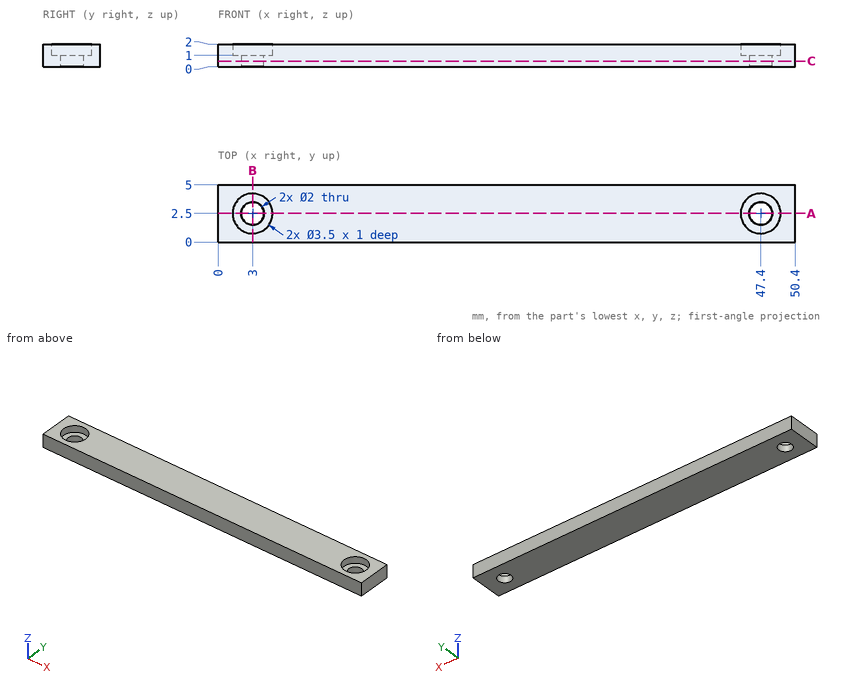
Answer from the drawing. Dimensions are ordinates in mm from the lowest x, y and z of the part. Coordinates: 2 decimals unless noted, no trailing zeros. Write each loop counter-clockwise with the first axis right and the second up, starting at its lowest first coordinate (ties: lowest second). Pieces come first, ordered by that corner, then holes. Notation, with made-up numbers: M -2,-36.5 L 15,-36.5 A29 ccw 15,-10.5 Z; hole C 22.5,80 d5. An arc over 180 degrees is marked long. Write item = value, one per line.
1. Straight lines are drawn through the part: line 1 (X direction, y = 2.5, z = 1.6); line 2 (X direction, y = 2.5, z = 0.65); line 3 (Y direction, x = 3, z = 1.3). For each, find the intervals that lie inside material, in ascending order. Write a range as from..to.
Solution:
line_1 = 0..1.25, 4.75..45.65, 49.15..50.4
line_2 = 0..2, 4..46.4, 48.4..50.4
line_3 = 0..0.75, 4.25..5
2. A flat-ended cylindrical pin translates along its axis: pin 1 (1.2 mm diameter, centred on x = 3, y = 2.5, fed in from +Z). Find the tip coordinate at first contact, or state that the pin passes through.
Solution:
pin_1 = through
3. The part is cut by section B-B (x = 3). Determine the outline of the cut face in (y, z), then the cut area to 3 significant figures.
Solution:
outline = M 0,0 L 1.5,0 L 1.5,1 L 0.75,1 L 0.75,2 L 0,2 Z; M 3.5,0 L 5,0 L 5,2 L 4.25,2 L 4.25,1 L 3.5,1 Z
area = 4.50 mm2
4. The part is cut by section C-C (z = 0.5). Determine the outline of the cut face in (x, y), then the cut area to 3 significant figures.
Solution:
outline = M 0,0 L 50.4,0 L 50.4,5 L 0,5 Z; hole C 3,2.5 d2; hole C 47.4,2.5 d2
area = 246 mm2
5. The part is cut by section A-A (y = 2.5). Determine the outline of the cut face in (x, z), then the cut area to 3 significant figures.
Solution:
outline = M 0,0 L 2,0 L 2,1 L 1.25,1 L 1.25,2 L 0,2 Z; M 4,0 L 46.4,0 L 46.4,1 L 45.65,1 L 45.65,2 L 4.75,2 L 4.75,1 L 4,1 Z; M 48.4,0 L 50.4,0 L 50.4,2 L 49.15,2 L 49.15,1 L 48.4,1 Z
area = 89.8 mm2
